For this review, use the dimensioned drawing (mm, ordinates from the lowest corner) and the shaded views. A direction names the side the tool comes from. Coordinates: 2 decimals unless noted, no trailing zeros. Write each loop counter-clockwise with the first axis right and the second up, starting at its lowest first coordinate (ties: lowest second). Pieces come first, ordered by that corner, then holes.
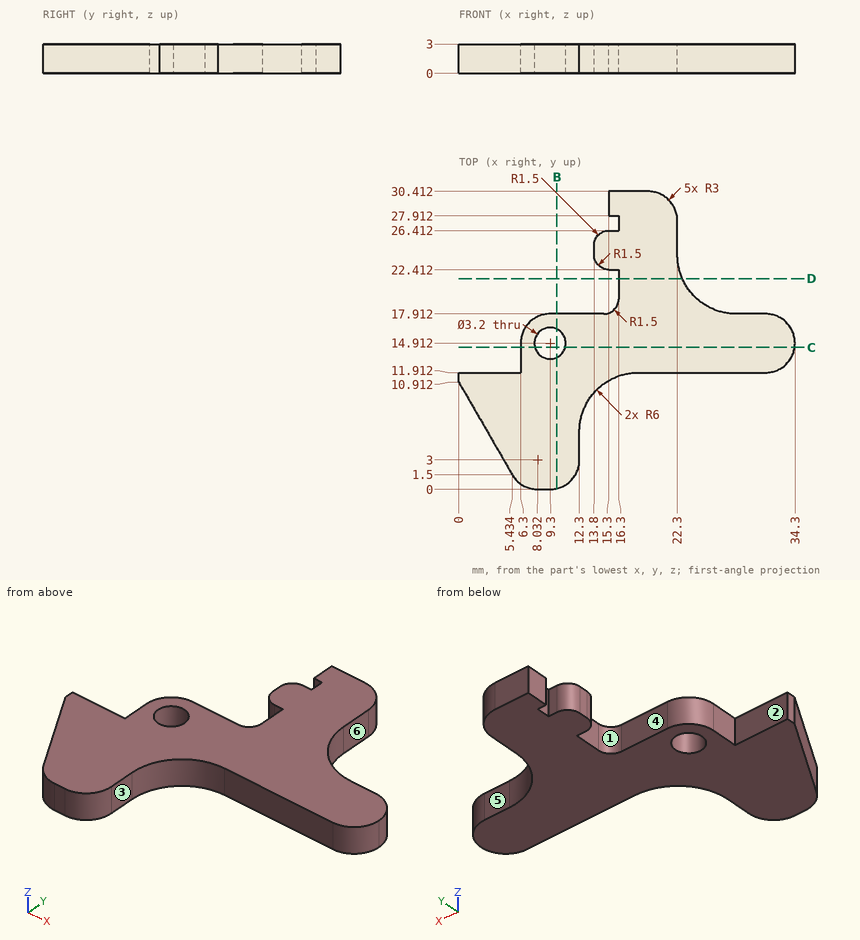
(1) For the marked faces 1, 2 and 3, list the 3-axis set-ups (+Z, -Z, +X, -X, +Y, -Y) from which the entire face can be reached by the end or side of a thin tool; tool diameter is ignored.
(2) Consider section D-D (y = 21.5). Give the boundary of the cut face in (x, z), plus the area to 3 significant figures.
(3) Wall thickness on line 1 (Y direction, x = 9.3, z = 1); line 2 (Y direction, x = 29, z = 0.75); line 3 (X direction, y = 14.5, z = 2.15): over which ranges is each line inside the solid? List them lowest first.
(4) Mouldability with a two-part tool opening along Y and no side actions: class the marked faces 4, 5 and 6 as +Y half, -Y half, draft (parallel to the pull), parting line (faces both ways), or undercut.
(5) Consider section B-B (x = 10). Give the boundary of the cut face in (y, z).
(6) Consider section C-C (y = 14.5). Give the boundary of the cut face in (x, z), plus the area to 3 significant figures.
(7) Insertion check: pin 1 Ø1.5 at (y, z) = (6, 2.5) entering from +X; pin 2 Ø3 at (x, y) = (9.3, 14.91) entering from -Z; pin 3 Ø1.1 at (x, z) = (15.5, 2) entering from -Y; pin 4 Ø1.5 at (x, z) = (29.5, 1.5) entering from +Y. Each pin has a flat end and moves straight along its axis. Give the tip position at first contact, or say it passes through.
Results:
1. face 1: +Z, -Z, -X
1. face 2: +Z, -Z, -X, +Y
1. face 3: +Z, -Z, +X, -Y
2. outline: (16.3, 0) - (22.81, 0) - (22.81, 3) - (16.3, 3) - close
2. area: 19.5 mm2
3. line 1: y = 0 to 13.31, 16.51 to 17.91
3. line 2: y = 11.91 to 17.91
3. line 3: x = 6.3 to 7.75, 10.85 to 34.27
4. face 4: undercut
4. face 5: +Y half
4. face 6: draft
5. outline: (0.08, 0) - (13.47, 0) - (13.47, 3) - (0.08, 3) - close; (16.35, 0) - (17.91, 0) - (17.91, 3) - (16.35, 3) - close
6. outline: (6.3, 0) - (7.75, 0) - (7.75, 3) - (6.3, 3) - close; (10.85, 0) - (34.27, 0) - (34.27, 3) - (10.85, 3) - close
6. area: 74.6 mm2
7. pin 1: stops at x = 12.36
7. pin 2: passes through
7. pin 3: stops at y = 10.89
7. pin 4: stops at y = 17.91
